The model under review builds one solid part; all positions refer to its coordinate system, in mm. A direction names the side the tool comes from. Give positions to 0.01 mm unless a question says otherwise; leave off trailing zeros. Order: outer loops, then holes, each group sorted by start corner. A loop starts at its lowest first (then second) coordinate and runs counter-clockwise, first axis right, second up.
```python
from build123d import *

# Parameters (mm, degrees)
F1_DEPTH        = 10
F2_SIZE         = 2
F4_D            = 1.2
F4_DEPTH        = 4
F4_TIP          = 0.3605163714
F4_COPIES_COUNT = 4


# Not quite as in the source:
# - a pattern or mirror of a feature is missing from the dataset's text; its kind, count and spacing are read off the source's solid


with BuildPart() as f1:
    # F0 (on Top) → F1 (new body, symmetric)
    with BuildSketch(Plane.XY):
        Polygon((8.5, 1.5), (-8.5, 1.5), (-8.5, -1.5), (8.5, -1.5), (8.5, -18.5), (11.5, -18.5), (11.5, 1.5), align=None)
    extrude(amount=F1_DEPTH, both=True)

    # F2
    f2_edges = [f1.edges().sort_by_distance(p)[0] for p in [
        (11.5, 1.5, 0),
    ]]
    chamfer(f2_edges, length=F2_SIZE)

    # F4
    with Locations(Plane.XZ.offset(1.5)):
        with Locations((-5, 0)):
            f4 = Hole(F4_D / 2, depth=F4_DEPTH)
            with Locations((0, 0, -(F4_DEPTH + F4_TIP / 2))):  # 118° drill point
                Cone(0, F4_D / 2, F4_TIP, mode=Mode.SUBTRACT)

    # F4_copies: F4 ×4 about axis
    f4_copies_axis = Axis((0, 0, 0), (0, 1, 0))
    for i in range(1, F4_COPIES_COUNT):
        add(f4.rotate(f4_copies_axis, i * 360 / F4_COPIES_COUNT), mode=Mode.SUBTRACT)


solid = f1.part
```
Item 1: For line 1 (Z direction, x = 5, y = 0.95); line 2 (X direction, y = -4.5, z = 2); line 3 (Y direction, x = 0.25, z = 8), list the stretches that pass through material, from the lowest coordinate up.
Values found:
line 1: z = -10 to -0.6, 0.6 to 10
line 2: x = 8.5 to 11.5
line 3: y = -1.5 to 1.5
Item 2: Take a section at D-D (z = 4). Give the boundary of the cut face in (x, y), and give its area (3 significant figures).
Values found:
outline: (-8.5, -1.5) - (8.5, -1.5) - (8.5, -18.5) - (11.5, -18.5) - (11.5, -0.5) - (9.5, 1.5) - (-8.5, 1.5) - close
area: 109 mm2
Item 3: Take a section at B-B (x = 0). Give the boundary of the cut face in (y, z), and give its area (3 significant figures).
Values found:
outline: (-1.5, -10) - (1.5, -10) - (1.5, -5.6) - (-1.5, -5.6) - close; (-1.5, -4.4) - (1.5, -4.4) - (1.5, 4.4) - (-1.5, 4.4) - close; (-1.5, 5.6) - (1.5, 5.6) - (1.5, 10) - (-1.5, 10) - close
area: 52.8 mm2
Item 4: Clearance check with flat-ended pins moving along their axes: pin 1 Ø3 at (x, y) = (7.5, -9.5) entering from -Z; pin 2 Ø4 at (y, z) = (-11, -2.5) entering from -X; pin 3 Ø2 at (x, z) = (6.5, 4) entering from -Y. State where each tip first meets the part, or that it passes through.
Values found:
pin 1: stops at z = -10
pin 2: stops at x = 8.5
pin 3: stops at y = -1.5
Item 5: For faces 1 (the flat face through (5, -1, -10)), 2 (the flat face through (8.5, -10, 0)), list the 3-axis set-ups (+Z, -Z, +X, -X, +Y, -Y) from which the entire face can be reached by the end or side of a thin tool; tool diameter is ignored.
Values found:
face 1: -Z, +X, -X, +Y, -Y
face 2: +Z, -Z, -X, -Y
Item 6: Draft analysis for pull direction X (two halves, no side actions). For faces 3 (the flat face through (5, -1, 10)), 4 (the flat face through (-8.5, 0, 0)), 5 (the cylindrical face through (-5.323, 0.021, 0.506)), state which applies: released by +X, released by -X, zero draft, split by the parting line, or undercut.
Values found:
face 3: zero draft
face 4: released by -X
face 5: undercut
Item 7: Take a section at A-A (z = -5). Give the boundary of the cut face in (x, y).
Values found:
outline: (-8.5, -1.5) - (-0.6, -1.5) - (-0.6, 1.5) - (-8.5, 1.5) - close; (0.6, -1.5) - (8.5, -1.5) - (8.5, -18.5) - (11.5, -18.5) - (11.5, -0.5) - (9.5, 1.5) - (0.6, 1.5) - close
Item 8: Take a section at C-C (x = -5). Give the boundary of the cut face in (y, z).
Values found:
outline: (-1.5, -10) - (1.5, -10) - (1.5, -0.6) - (-1.5, -0.6) - close; (-1.5, 0.6) - (1.5, 0.6) - (1.5, 10) - (-1.5, 10) - close
